```python
from build123d import *

# Parameters (mm, degrees)
SKETCH1_W             = 15.25
SKETCH1_H             = 20
SKETCH1_R             = 2.25
BOSS_EXTRUDE1_DEPTH   = 3
BOSS_EXTRUDE1_2_DEPTH = 3
SKETCH2_W             = 45.5
SKETCH2_H             = 3
BOSS_EXTRUDE2_DEPTH   = 42
SKETCH3_R             = 8.25
CUT_EXTRUDE1_DEPTH    = 61.44447165
BOSS_EXTRUDE3_DEPTH   = 2
LPATTERN1_COUNT       = 2
LPATTERN1_PITCH       = 43.5
CUT_EXTRUDE2_DEPTH    = 61.44447165
BOSS_EXTRUDE4_DEPTH   = 3
CUT_EXTRUDE3_DEPTH    = 61.44447165
SKETCH10_W            = 10
SKETCH10_H            = 2.5
CUT_EXTRUDE4_DEPTH    = 2
BOSS_EXTRUDE5_REACH   = 66.609
SKETCH13_W            = 3
SKETCH13_H            = 11.133974596
CUT_EXTRUDE6_DEPTH    = 1
CHAMFER1_SIZE         = 1
BOSS_EXTRUDE6_DEPTH   = 13.25
CHAMFER2_SIZE         = 1


with BuildPart() as part:
    # Sketch1 → Boss-Extrude1 (new body)
    with BuildSketch(Plane.XY):
        with Locations((-28.974646897, 6.034741944)):
            Rectangle(SKETCH1_W, SKETCH1_H)
        with Locations((-29.599646897, 6.034741944)):
            Circle(SKETCH1_R, mode=Mode.SUBTRACT)
    extrude(amount=BOSS_EXTRUDE1_DEPTH)


with BuildPart() as body_2:
    # Sketch1 → Boss-Extrude1 2 (new body)
    with BuildSketch(Plane.XY):
        with Locations((1.275353103, 6.034741944)):
            Rectangle(SKETCH1_W, SKETCH1_H)
        with Locations((1.900353103, 6.034741944)):
            Circle(SKETCH1_R, mode=Mode.SUBTRACT)
    extrude(amount=BOSS_EXTRUDE1_2_DEPTH)



with BuildPart() as body_3:
    # Sketch2 → Boss-Extrude2 (new body)
    with BuildSketch(Plane.XY.offset(3)):
        with Locations((-13.849646897, 14.534741944)):
            Rectangle(SKETCH2_W, SKETCH2_H)
    extrude(amount=BOSS_EXTRUDE2_DEPTH)

    # Sketch3 → Cut-Extrude1 (cut, through all)
    with BuildSketch(Plane(origin=(0, 13.034741944, 0), x_dir=(-1, 0, 0), z_dir=(0, -1, 0))):
        with Locations(Location((26.924646897, -35, 0), (0, 0, 90))):
            Circle(SKETCH3_R)
        with Locations(Location((0.774646897, -35, 0), (0, 0, 90))):
            Circle(SKETCH3_R)
    extrude(amount=-CUT_EXTRUDE1_DEPTH, mode=Mode.SUBTRACT)


with BuildPart() as body_2_1:
    add(body_2.part)

    add(body_3.part)  # Boss-Extrude3 merges body 3
    # Sketch4 → Boss-Extrude3 (add)
    with BuildSketch(Plane(origin=(8.900353103, 0, 0), x_dir=(0, 0, -1), z_dir=(1, 0, 0))):
        Polygon((-3, -3.965258056), (-24, 13.034741944), (-3, 13.034741944), align=None)
    boss_extrude3 = extrude(amount=-BOSS_EXTRUDE3_DEPTH)


with BuildPart() as part_1:
    add(part.part)

    add(body_2_1.part)  # LPattern1 merges body 2
    # LPattern1: Boss-Extrude3 ×2
    with Locations(*[(-i * LPATTERN1_PITCH, 0, 0) for i in range(1, LPATTERN1_COUNT)]):
        add(boss_extrude3)

    # Sketch5 → Cut-Extrude2 (cut, through all)
    with BuildSketch(Plane(origin=(0, 13.034741944, 0), x_dir=(-1, 0, 0), z_dir=(0, -1, 0))):
        Polygon((29.424646897, -8), (29.424646897, -25.5), (24.424646897, -25.5), (24.424646897, -8), (25.424646897, -8), (25.424646897, -24.5), (28.424646897, -24.5), (28.424646897, -8), align=None)
        Polygon((-0.725353103, -8), (-1.725353103, -8), (-1.725353103, -25.5), (3.274646897, -25.5), (3.274646897, -8), (2.274646897, -8), (2.274646897, -24.5), (-0.725353103, -24.5), align=None)
    extrude(amount=-CUT_EXTRUDE2_DEPTH, mode=Mode.SUBTRACT)

    # Sketch6 → Boss-Extrude4 (add)
    with BuildSketch(Plane(origin=(-25.424646897, 0, 0), x_dir=(0, 0, -1), z_dir=(1, 0, 0))):
        Polygon((-24.5, 13.034741944), (-26, 12.16871654), (-26, 10.66871654), (-21.5, 10.66871654), (-19.133974596, 13.034741944), align=None)
    boss_extrude4 = extrude(amount=-BOSS_EXTRUDE4_DEPTH)

    # Mirror7: Boss-Extrude4 across plane
    add(boss_extrude4.mirror(Plane(origin=(-13.849646897, 13.034741944, 8), x_dir=(0, 0, 1), z_dir=(1, 0, 0))))

    # Sketch9 → Cut-Extrude3 (cut, through all)
    with BuildSketch(Plane(origin=(0, 13.034741944, 0), x_dir=(-1, 0, 0), z_dir=(0, -1, 0))):
        with BuildLine():
            Line((16.849646897, -45), (10.849646897, -45))
            ThreePointArc((10.849646897, -45), (8.099646897, -42.25), (10.849646897, -39.5))
            Line((10.849646897, -39.5), (16.849646897, -39.5))
            ThreePointArc((16.849646897, -39.5), (19.599646897, -42.25), (16.849646897, -45))
        make_face()
    extrude(amount=-CUT_EXTRUDE3_DEPTH, mode=Mode.SUBTRACT)

    # Sketch10 → Cut-Extrude4 (cut)
    with BuildSketch(Plane(origin=(0, 13.034741944, 0), x_dir=(-1, 0, 0), z_dir=(0, -1, 0))):
        with Locations((13.849646897, -26.25)):
            Rectangle(SKETCH10_W, SKETCH10_H)
    extrude(amount=-CUT_EXTRUDE4_DEPTH, mode=Mode.SUBTRACT)

    # Boss-Extrude5: up to this face of the body (flat: up to its plane)
    boss_extrude5_end = Plane(part_1.part.faces().sort_by_distance((6.900353103, 7.368075277, 10))[0])
    # Sketch11 → Boss-Extrude5 (add, up to the picked face)
    with BuildSketch(Plane(origin=(-34.599646897, 0, 0), x_dir=(0, 0, -1), z_dir=(1, 0, 0)), mode=Mode.PRIVATE) as boss_extrude5_sk1:
        Polygon((-5.617808219, -1.846079974), (-3, -3.965258056), (-3, -0.465258056), (-4.5, -0.465258056), align=None)
    boss_extrude5_tool1 = split(extrude(boss_extrude5_sk1.sketch, amount=BOSS_EXTRUDE5_REACH, mode=Mode.PRIVATE), bisect_by=boss_extrude5_end, keep=Keep.BOTH, mode=Mode.PRIVATE)
    add(boss_extrude5_tool1.solids().sort_by(Axis((-34.599647, -1.87709, 3.964792), (1, 0, 0)))[0])

    # Sketch13 → Cut-Extrude6 (cut)
    with BuildSketch(Plane(origin=(0, 13.034741944, 0), x_dir=(-1, 0, 0), z_dir=(0, -1, 0))):
        with Locations((26.924646897, -13.566987298)):
            Rectangle(SKETCH13_W, SKETCH13_H)
        with Locations((0.774646897, -13.566987298)):
            Rectangle(SKETCH13_W, SKETCH13_H)
    extrude(amount=-CUT_EXTRUDE6_DEPTH, mode=Mode.SUBTRACT)

    # Chamfer1
    chamfer1_edges = [part_1.edges().sort_by_distance(p)[0] for p in [
        (-26.924646897, 14.034741944, 8),
        (-0.774646897, 14.034741944, 8),
    ]]
    chamfer(chamfer1_edges, length=CHAMFER1_SIZE - 0.0001)  # a hair under: the kernel refuses the full size

    # Sketch11<3> → Boss-Extrude6 (add)
    with BuildSketch(Plane(origin=(-34.599646897, 0, 0), x_dir=(0, 0, -1), z_dir=(1, 0, 0))):
        Polygon((-4.5, -0.465258056), (-3, -0.465258056), (-3, 1.38768312), align=None)
    boss_extrude6 = extrude(amount=BOSS_EXTRUDE6_DEPTH)

    # Mirror8: Boss-Extrude6 across plane
    add(boss_extrude6.mirror(Plane(origin=(-13.849646897, 13.034741944, 8), x_dir=(0, 0, 1), z_dir=(1, 0, 0))))

    # Chamfer2
    chamfer2_edges = [part_1.edges().sort_by_distance(p)[0] for p in [
        (-28.424646897, 14.534791944, 8),
        (-2.274646897, 14.534791944, 8),
        (-25.424646897, 14.534791944, 8),
        (0.725353103, 14.534791944, 8),
    ]]
    chamfer(chamfer2_edges, length=CHAMFER2_SIZE - 0.0001)  # a hair under: the kernel refuses the full size


solid = part_1.part
```
Design review of the part built by this model. Coordinates are the model's own, in mm. A direction names the side the tool comes from. Coordinates: 2 decimals unless noted, no trailing zeros. Order: outer loops, then holes, each group sorted by start corner. A loop starts at its lowest first (then second) coordinate and runs counter-clockwise, first axis right, second up. Notation, with made-up numbers: M 47,-9 L 66,-9 A13 ccw 66,5 Z; hole C 71.5,39.5 d2. An arc over 180 degrees is marked long. Answer as a JSON object with one key per item and string values. Group by question number.
1) For pin 1 (0.9 mm diameter, centred on x = -12.5, y = 14, fed in from -Z); pin 2 (1.2 mm diameter, centred on x = -1, y = 11.5, fed in from +Z); pin 3 (1.5 mm diameter, centred on x = -27.5, z = 12, fed in from -Y), all flat-tipped, find the tip position at first contact; note any pin that passes through.
2) Tool access review of faces 1 (the flat face through (-1, 10.669, 24)), 2 (the flat face through (-1, 15, 24.5)), 3 (the flat face through (-27, 14.035, 14)), 4 (the flat face through (1.725, 15, 17)): name each direction out of +Z, -Z, +X, -X, +Y, -Y from which nothing blocks a thin tool from reaching the whole face with its end or side.
3) Add section D-D, the plane y = 2.5. Write out the cut boundary in (x, z).
4) Add section C-C, the plane z = 23. Write out the cut boundary in (x, y).
5) Mouldability with a two-part tool opening along X and no side actions: class faces 5 (the flat face through (8.9, 8, 12)), 6 (the flat face through (-27, 10.669, 24)), 7 (the flat face through (-27, 15, 24.5)) as pulls with the +X half, pulls with the -X half, needs draft (parallel to the pull), parting line crosses it, or undercut.
6) Add section B-B, the plane y = 11.5. Write out the cut boundary in (x, z).
7) Wall thickness on L1, parallel to X at y = 14.5, z = 34; L2, parallel to X at y = 12, z = 23; L3, parallel to Z at x = -16.5, y = 13.5: over which ranges is each line inside the solid? List them lowest first.
8) Add section A-A, the plane z = 35. Write out the cut boundary in (x, y).
Computed values:
{
 "1": {"pin 1": "stops at z = 3", "pin 2": "stops at z = 26", "pin 3": "stops at y = 14.03"},
 "2": {"face 1": "+Z, +X, -X, -Y", "face 2": "+Y", "face 3": "-Y", "face 4": "+Y, -Y"},
 "3": {"outline": "M -36.6,0 L -21.35,0 L -21.35,3 L -34.6,3 L -34.6,10.99 L -36.6,10.99 Z; M -6.35,0 L 8.9,0 L 8.9,10.99 L 6.9,10.99 L 6.9,3 L -6.35,3 Z"},
 "4": {"outline": "M -36.6,12.23 L -34.6,12.23 L -34.6,13.03 L -29.42,13.03 L -29.42,16.03 L -36.6,16.03 Z; M -28.42,10.67 L -25.42,10.67 L -25.42,16.03 L -28.42,16.03 Z; M -24.42,13.03 L -3.27,13.03 L -3.27,16.03 L -24.42,16.03 Z; M -2.27,10.67 L 0.73,10.67 L 0.73,16.03 L -2.27,16.03 Z; M 1.73,13.03 L 6.9,13.03 L 6.9,12.23 L 8.9,12.23 L 8.9,16.03 L 1.73,16.03 Z"},
 "5": {"face 5": "pulls with the +X half", "face 6": "needs draft", "face 7": "undercut"},
 "6": {"outline": "M -36.6,0 L -21.35,0 L -21.35,3 L -34.6,3 L -34.6,22.1 L -36.6,22.1 Z; M -28.42,20.67 L -25.42,20.67 L -25.42,26 L -28.42,26 Z; M -6.35,0 L 8.9,0 L 8.9,22.1 L 6.9,22.1 L 6.9,3 L -6.35,3 Z; M -2.27,20.67 L 0.73,20.67 L 0.73,26 L -2.27,26 Z"},
 "7": {"L1": "x = -36.6 to -35.11, -18.74 to -8.96, 7.41 to 8.9", "L2": "x = -28.42 to -25.42, -2.27 to 0.73", "L3": "z = 3 to 25, 27.5 to 39.5"},
 "8": {"outline": "M -36.6,13.03 L -35.17,13.03 L -35.17,16.03 L -36.6,16.03 Z; M -18.67,13.03 L -9.02,13.03 L -9.02,16.03 L -18.67,16.03 Z; M 7.48,13.03 L 8.9,13.03 L 8.9,16.03 L 7.48,16.03 Z"}
}
